Verification items for the finished model (mm, model axes). Face numbers are marked on the shaded views. A direction names the side the tool comes from. Round coordinates to 2 decimals unless told otherwise and drop trailing zeros. Order: outer loops, then holes, each group sorted by start corner. A loop starts at its lowest first (then second) coordinate and runs counter-clockwise, first axis right, second up.
Autodesk Inventor part; units mm, degrees
ref_plane "YZ Plane" through (0, 0, 0) normal (1, 0, 0) x (0, 1, 0)
ref_plane "XZ Plane" through (0, 0, 0) normal (0, 1, 0) x (-1, 0, 0)
ref_plane "XY Plane" through (0, 0, 0) normal (0, 0, 1) x (1, 0, 0)
sketch "Sketch1" plane through (0, 0, 0) normal (0, 0, 1) x (1, 0, 0)
  line L0 (0, 0) -> (0, 8) construction
  line L1 (6, 0) -> (12.5, 0)
  line L2 (12.5, 0) -> (12.5, 2)
  line L3 (12.5, 2) -> (8.5, 2)
  line L4 (8.5, 2) -> (8.5, 8)
  line L5 (8.5, 8) -> (6, 8)
  line L6 (6, 8) -> (6, 3)
  line L7 (6, 3) -> (5.25, 3)
  line L8 (5.25, 3) -> (5.25, 0)
  line L9 (5.25, 0) -> (6, 0)
  line L10 (6, 0) -> (6, 0)
  line L11 (10.5, 2) -> (10.5, 0) construction
  line L12 (9.5, 2) -> (11.5, 2) construction
  line L13 (11.5, 2) -> (11.5, 0) construction
  line L14 (11.5, 0) -> (9.5, 0) construction
  line L15 (9.5, 0) -> (9.5, 2) construction
  line L16 (9.5, 2) -> (11.5, 0) construction
  line L17 (11.5, 2) -> (9.5, 0) construction
  line L18 (-2.5, 0) -> (15, 0) construction
  point P0 (10.5, 1)
  dimension "d1" = 2
  dimension "d3" = 2
  dimension "d4" = 12
  dimension "d5" = 2.5
  dimension "JointFixation_FixHole_Dia" = 21
  dimension "ShaftFixation_UpperLower_Height" = 8
  dimension "Bearing_OuterRing_Dia" = 10.5
  dimension "JointFixation_DiaOut" = 25
  dimension "d28" = 5
revolve "Revolution1" add sketch "Sketch1" angle 360 about axis through (0, 0, 0) along (0, 1, 0)
sketch "Sketch2" plane through (0, 2, 0) normal (0, 1, 0) x (1, 0, 0)
  circle A0 centre (0, 0) radius 8.5
  circle A1 centre (0, 0) radius 12.5
  line L0 (-9.1652, 8.5) -> (9.1652, 8.5)
  line L1 (-9.1652, -8.5) -> (9.1652, -8.5)
  circle A2 centre (0, 0) radius 10.5 construction
  line L2 (0, 0) -> (-10.5, 0) construction
  point P0 (0, 0)
  point P1 (10.5, 0)
  dimension "d14" = 21
  dimension "d17" = 360
  dimension "LowerArm_BearingFixFlansch_Width" = 17
hole "Hole1" at (-10.5, 2, 0) at (10.5, 2, 0) direction (0, -1, 0) diameter 1.567 end through all
equation "\"d14\" = JointFixation_FixHole_Dia"
properties part number "LowerArm_JointFixation" material "Aluminum 6061"
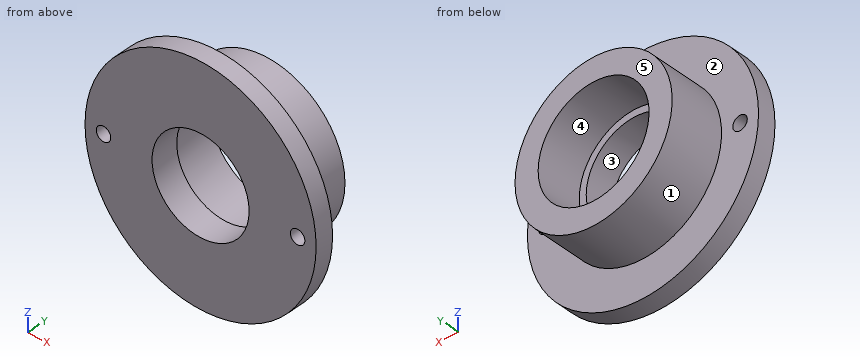
1) Go/stop test with flat-tipped pins: pin 1 Ø9.5 at (x, z) = (0, 0) entering from +Y; pin 2 Ø3 at (y, z) = (7, -3) entering from -X; pin 3 Ø4 at (y, z) = (2, 6.5) entering from -X. Record where each tip stops, or that it passes through.
2) Sectioned sample at B-B on z = 0. Record the cut outline in (x, y).
3) Scan lines: probe 1 along X at (y, z) = (4.6, 0); probe 2 along X at (y, z) = (1.4, 0); probe 3 along Z at (x, y) = (0, 2.35). Record each from-to range of solid material in increasing order.
4) Sectioned sample at A-A on x = 0. Record the cut outline in (y, z).
5) Draft check along Z on the marked faces 1, 2 and 3. Enter one of: released by +Z, released by -Z, zero draft, split by the parting line, or undercut.
6) Tool access check on the marked faces 4 and 5. Record the directions out of +Z, -Z, +X, -X, +Y, -Y that give a thin tool (end or side, any length) a straight path to the whole face; none if there is none.
7) Sectioned sample at C-C on y = 1. Record the cut outline in (x, z).
8) Sectioned sample at D-D on z = 3.5. Record the cut outline in (x, y).
Returned:
1. pin 1: passes through
1. pin 2: stops at x = -8.37
1. pin 3: stops at x = -11.66
2. outline: (-12.5, 0) - (-11.28, 0) - (-11.28, 2) - (-12.5, 2) - close; (-9.72, 0) - (-5.25, 0) - (-5.25, 3) - (-6, 3) - (-6, 8) - (-8.5, 8) - (-8.5, 2) - (-9.72, 2) - close; (5.25, 0) - (9.72, 0) - (9.72, 2) - (8.5, 2) - (8.5, 8) - (6, 8) - (6, 3) - (5.25, 3) - close; (11.28, 0) - (12.5, 0) - (12.5, 2) - (11.28, 2) - close
3. probe 1: x = -8.5 to -6, 6 to 8.5
3. probe 2: x = -12.5 to -11.28, -9.72 to -5.25, 5.25 to 9.72, 11.28 to 12.5
3. probe 3: z = -8.5 to -5.25, 5.25 to 8.5
4. outline: (0, -12.5) - (2, -12.5) - (2, -8.5) - (8, -8.5) - (8, -6) - (3, -6) - (3, -5.25) - (0, -5.25) - close; (0, 5.25) - (3, 5.25) - (3, 6) - (8, 6) - (8, 8.5) - (2, 8.5) - (2, 12.5) - (0, 12.5) - close
5. face 1: split by the parting line
5. face 2: zero draft
5. face 3: undercut
6. face 4: +Y
6. face 5: +Z, -Z, +X, -X, +Y
7. outline: circle Ø25 at (0, 0); hole circle Ø1.57 at (-10.5, 0); hole circle Ø10.5 at (0, 0); hole circle Ø1.57 at (10.5, 0)
8. outline: (-12, 0) - (-3.91, 0) - (-3.91, 3) - (-4.87, 3) - (-4.87, 8) - (-7.75, 8) - (-7.75, 2) - (-12, 2) - close; (3.91, 0) - (12, 0) - (12, 2) - (7.75, 2) - (7.75, 8) - (4.87, 8) - (4.87, 3) - (3.91, 3) - close
